Autodesk Inventor part; units mm, degrees
ref_plane "YZ Plane" through (0, 0, 0) normal (1, 0, 0) x (0, 1, 0)
ref_plane "XZ Plane" through (0, 0, 0) normal (0, 1, 0) x (-1, 0, 0)
ref_plane "XY Plane" through (0, 0, 0) normal (0, 0, 1) x (1, 0, 0)
sketch "Sketch1" plane through (0, 0, 0) normal (0, 0, 1) x (1, 0, 0)
  line L0 (-9.2616, -16.795) -> (16.1384, -16.795)
  line L1 (16.1384, -16.795) -> (16.1384, 2.255)
  line L2 (16.1384, 2.255) -> (-10.4396, 25.877)
  line L3 (-10.4396, 25.877) -> (-32.2486, 25.877)
  line L4 (-32.2486, 25.877) -> (-32.2486, 10.891)
  line L5 (-32.2486, 10.891) -> (-9.2616, 10.891)
  line L6 (-9.2616, -16.795) -> (-9.2616, 10.891)
  dimension "d39" = 25.4
  dimension "d40" = 22.987
  dimension "d42" = 27.686
  dimension "d43" = 14.986
  dimension "d45" = 48.37
  dimension "d46" = 19.05
extrude "Extrusion1" add sketch "Sketch1" along normal blind 63.5
sketch "Sketch5" plane through (16.1384, -16.795, 0) normal (1, 0, 0) x (0, 0, -1)
  line L0 (0, 0) -> (-63.5, 0)
  line L1 (-63.5, 0) -> (-63.5, 19.05)
  line L2 (-63.5, 0) -> (-52.07, 12.7) construction
  line L3 (-52.07, 12.7) -> (-11.43, 12.7) construction
  line L4 (0, 0) -> (0, 19.05) construction
  line L5 (-11.43, 12.7) -> (0, 0) construction
  point P0 (0, 16.795)
  dimension "d47" = 12.7
  dimension "d48" = 11.43
hole "Hole3" at (16.1384, -4.095, 52.07) at (16.1384, -4.095, 11.43) direction (-1, 0, 0) diameter 6.7564 end through all counterbore diameter 19.05 counterbore depth 9.525
fillet "Fillet2" radius 3.175 7 edges at (16.1384, 2.255, 31.75) (16.1384, 2.255, 61.3348) (16.1384, 2.255, 2.1652) (16.1384, -16.795, 31.75) (-9.2616, -16.795, 31.75) (-10.4396, 25.877, 31.75) (-32.2486, 25.877, 31.75)
properties part number "C29_TK_BackWedge" material "ABS Plastic"
Verification items for the finished model (mm, model axes). A direction names the side the tool comes from. Coordinates: 2 decimals unless noted, no trailing zeros. Order: outer loops, then holes, each group sorted by start corner. A loop starts at its lowest first (then second) coordinate and runs counter-clockwise, first axis right, second up. Notation, with made-up numbers: (-37.5, 65) -> (7.5, 65) arc R14 ccw to (7.5, 76) -> close; hole circle Ø3 at (60.25, -4.75). An arc over 180 degrees is marked (long way). Put each result on its own line as item: value. Start each with the question number.
1. Material ranges on L1, parallel to Z at x = 9, y = -2.5; L2, parallel to X at y = -10, z = 8.5; L3, parallel to Z at x = 3.5, y = -5, recorded low to high. Write a range as [from, to].
2. Cross-section at C-C, the plane y = -2. Record the boundary of the cut face in (x, z), then the cut area to 3 significant figures.
3. Mould release check, pull along Z, two halves, no side actions. Record for faces 1 (the cylindrical face through (-1.435, -5.11, 8.208)), 2 (the flat face through (-3, 5, 63.5)), 3 (the flat face through (-32.249, 17, 31)): released by +Z, released by -Z, zero draft, split by the parting line, or undercut.
4. Cross-section at D-D, the plane x = 3. Record the boundary of the cut face in (y, z) (3 decimals).
5. Go/stop test with flat-tipped pins: pin 1 Ø11 at (y, z) = (-4.095, 52.07) entering from -X; pin 2 Ø6 at (y, z) = (-4.095, 11.43) entering from -X; pin 3 Ø2 at (x, z) = (-14.5, 40.5) entering from -Y; pin 4 Ø3 at (x, z) = (-7.5, 52.5) entering from +Y. Record where each tip stops, or that it passes through.
6. Access from +Z, -Z, +X, -X, +Y, -Y to the whole of each face (thin tool, end or side, straight path). Record for faces 4 (the flat face through (-9.262, -2, 31)), 5 (the flat face through (6.613, 0, 52)), 6 (the cylindrical face through (15.87, 2.11, 2.1)).
7. Cross-section at B-B, the plane z = 36. Record the boundary of the cut face in (x, y) (1 decimal), then the cut area to 3 significant figures.
Computed:
1. L1: [0, 2.04], [20.82, 42.68], [61.46, 63.5]
1. L2: [-9.26, 6.61]
1. L3: [0, 8.18], [14.68, 48.82], [55.32, 63.5]
2. outline: (-9.26, 0) -> (16.14, 0) -> (16.14, 2.14) -> (6.61, 2.14) -> (6.61, 8.78) -> (-9.26, 8.78) -> close; (-9.26, 14.08) -> (6.61, 14.08) -> (6.61, 20.72) -> (16.14, 20.72) -> (16.14, 42.78) -> (6.61, 42.78) -> (6.61, 49.42) -> (-9.26, 49.42) -> close; (-9.26, 54.72) -> (6.61, 54.72) -> (6.61, 61.36) -> (16.14, 61.36) -> (16.14, 63.5) -> (-9.26, 63.5) -> close
2. area: 1,090 mm2
3. face 1: undercut
3. face 2: released by +Z
3. face 3: zero draft
4. outline: (-16.795, 0) -> (13.932, 0) -> (13.932, 63.5) -> (-16.795, 63.5) -> close; hole circle Ø6.756 at (-4.095, 11.43); hole circle Ø6.756 at (-4.095, 52.07)
5. pin 1: x = -9.26
5. pin 2: through
5. pin 3: y = 10.89
5. pin 4: y = 24.6
6. face 4: +Z, -Z, -X, -Y
6. face 5: +X
6. face 6: +Z, -Z, +X, +Y
7. outline: (-32.2, 10.9) -> (-9.3, 10.9) -> (-9.3, -13.6) arc R3.2 ccw to (-6.1, -16.8) -> (13, -16.8) arc R3.2 ccw to (16.1, -13.6) -> (16.1, 0.8) arc R3.2 ccw to (15.1, 3.2) -> (-9.5, 25.1) arc R3.2 ccw to (-11.6, 25.9) -> (-29.1, 25.9) arc R3.2 ccw to (-32.2, 22.7) -> close
7. area: 1,110 mm2
